```python
from build123d import *

# Parameters (mm, degrees)
F0_W     = 76.2
F0_H     = 50.8
F1_DEPTH = 25.4
F2_W     = 70.472512
F2_H     = 38.386009
F3_DEPTH = 20.32
F4_R     = 1.164425
F4_R_2   = 1.122016
F4_R_3   = 1.274708
F4_R_4   = 1.273834
F5_DEPTH = 20.32


with BuildPart() as f1:
    # F0 (on Top) → F1 (new body)
    with BuildSketch(Plane.XY):
        with Locations((38.1, 25.4)):
            Rectangle(F0_W, F0_H)
    extrude(amount=-F1_DEPTH)

    # F2 (on Top) → F3 (cut)
    with BuildSketch(Plane.XY):
        with Locations((37.732361, 25.370613)):
            Rectangle(F2_W, F2_H)
    extrude(amount=-F3_DEPTH, mode=Mode.SUBTRACT)

    # F4 (on Top) → F5 (join)
    with BuildSketch(Plane.XY):
        with Locations((3.776019, 46.978962)):
            Circle(F4_R)
        with Locations((72.362818, 46.967924)):
            Circle(F4_R_2)
        with Locations((72.392121, 3.830065)):
            Circle(F4_R_3)
        with Locations((3.809462, 3.828035)):
            Circle(F4_R_4)
    extrude(amount=F5_DEPTH)


solid = f1.part
```
Here's how the part is built. I have some questions about the finished solid (model axes, mm). A direction names the side the tool comes from. Coordinates: 2 decimals unless noted, no trailing zeros. Order: outer loops, then holes, each group sorted by start corner. A loop starts at its lowest first (then second) coordinate and runs counter-clockwise, first axis right, second up.
1) Which directions (+Z, -Z, +X, -X, +Y, -Y) give clear straight access to the entire face, cutting with the end or side of a thin tool? Please do faces 1 (the face through (76.2, 25, -13)), 2 (the face through (72.22, 48.08, 10.02)).
2) We'd pull the mould along X, two halves only. Please class faces 3 (the face through (0, 25, -13)), 4 (the face through (72.969, 25, -10)), 5 (the face through (4, 4, 20.32)): +X half, -X half, draft (parallel to the pull), parting line (faces both ways), or undercut.
3) I need wall thicknesses on line 1 (Y direction, x = 61, z = -11); line 2 (X direction, y = 22.5, z = -10.5); line 3 (Z direction, x = 32, y = 3.5). Which ranges of each line are inside material? Lowest first, please.
4) Imagine slicing it at B-B on x = 13. List the corners of the cut face in (y, z) for me, and give its area (3 significant figures).
5) Imagine slicing it at A-A on z = -5. List the corners of the cut face in (x, y) for me, and give its area (3 significant figures).
6) Imagine slicing it at D-D on z = 7. List the corners of the cut face in (x, y) for me, and give its area (3 significant figures).
7) Will these pins go through, and if not, where does the flat tip stop? pin 1 (3 mm diameter, centred on x = 12.5, y = 43.5, fed in from +Z); pin 2 (11.5 mm diameter, centred on x = 40.5, y = 22.5, fed in from +Z).
8) Imagine slicing it at C-C on y = 17. List the corners of the cut face in (x, z) for me, and give its area (3 significant figures).
Response values:
1. face 1: +Z, -Z, +X, +Y, -Y
1. face 2: +Z
2. face 3: -X half
2. face 4: undercut
2. face 5: draft
3. line 1: y = 0 to 6.18, 44.56 to 50.8
3. line 2: x = 0 to 2.5, 72.97 to 76.2
3. line 3: z = -25.4 to 0
4. outline: (0, -25.4) - (50.8, -25.4) - (50.8, 0) - (44.56, 0) - (44.56, -20.32) - (6.18, -20.32) - (6.18, 0) - (0, 0) - close
4. area: 510 mm2
5. outline: (0, 0) - (76.2, 0) - (76.2, 50.8) - (0, 50.8) - close; hole (2.5, 6.18) - (72.97, 6.18) - (72.97, 44.56) - (2.5, 44.56) - close
5. area: 1,170 mm2
6. outline: circle Ø2.55 at (3.81, 3.83); circle Ø2.33 at (3.78, 46.98); circle Ø2.55 at (72.39, 3.83); circle Ø2.24 at (72.36, 46.97)
6. area: 18.4 mm2
7. pin 1: stops at z = 0
7. pin 2: stops at z = -20.32
8. outline: (0, -25.4) - (76.2, -25.4) - (76.2, 0) - (72.97, 0) - (72.97, -20.32) - (2.5, -20.32) - (2.5, 0) - (0, 0) - close
8. area: 503 mm2
